The listing builds one solid part. Answer for the finished solid, in the listing's coordinates (mm). Coordinates: 2 decimals unless noted, no trailing zeros. Loops run counter-clockwise (first coordinate to the right, second up) from the corner with the lowest first, then second, coordinate; pieces in that order, holes last. Notation, with made-up numbers: M 2.25,9.5 L 50.25,9.5 A22 cw 50.25,41.5 Z; hole C 15.25,47 d6. An arc over 180 degrees is marked long. Answer as a JSON object with one key per item and string values. Group by question number.
1. A cutting plane is placed at D-D on x = 25. Give the vertices of the cut face in (y, z).
2. A cutting plane is placed at C-C on x = -5. Give the vertices of the cut face in (y, z), and give its area (3 significant figures).
3. Straight lines are drawn through the part: L1, parallel to Y at x = -42.5, z = 1.75; L2, parallel to X at y = -6.5, z = 2.75; L3, parallel to Y at x = -45, z = 0.45. For each, find the intervals that lie inside material, in ascending order.
4. Given pin 1 (1.5 mm diameter, centred on y = -7, z = 1.5, fed in from -X); pin 2 (1.5 mm diameter, centred on y = -7.5, z = 1, fed in from +X), each flat-ended and moving along its own axis, determine where each tip first touches the part or whether it passes through.
5. A cutting plane is placed at A-A on z = 0.8. State how many separate pieces and enclosed holes the cut face has, and give its area (3 significant figures).
6. A cutting plane is placed at B-B on x = -49.5. Give the vertices of the cut face in (y, z), and give its area (3 significant figures).
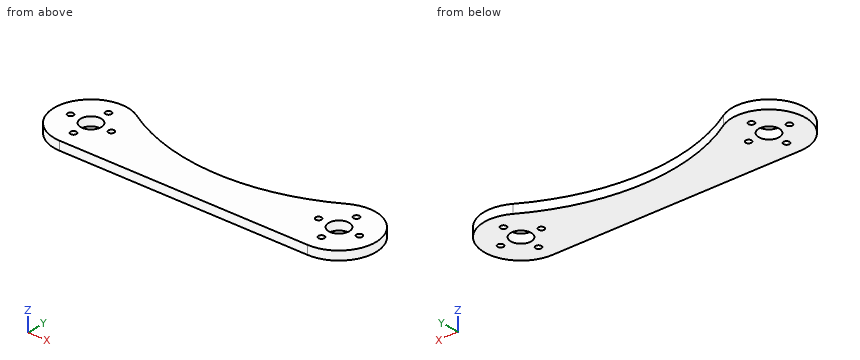
from build123d import *

# Parameters (mm, degrees)
SKETCH1_R           = 3.5
SKETCH1_R_2         = 1
BOSS_EXTRUDE1_DEPTH = 3


with BuildPart() as part:
    # Sketch1 → Boss-Extrude1 (new body)
    with BuildSketch(Plane.XY):
        with BuildLine():
            Line((-42.5, -12.5), (42.5, -12.5))
            ThreePointArc((42.5, -12.5), (54.545159585, 3.341276787), (36.060606061, 10.713739109))
            ThreePointArc((36.060606061, 10.713739109), (0, 0.710678119), (-36.060606061, 10.713739109))
            ThreePointArc((-36.060606061, 10.713739109), (-54.545159585, 3.341276787), (-42.5, -12.5))
        make_face()
        with Locations((-42.5, 0)):
            Circle(SKETCH1_R, mode=Mode.SUBTRACT)
        with Locations((42.5, 0)):
            Circle(SKETCH1_R, mode=Mode.SUBTRACT)
        with Locations((-42.5, 7)):
            Circle(SKETCH1_R_2, mode=Mode.SUBTRACT)
        with Locations((-35.5, 0)):
            Circle(SKETCH1_R_2, mode=Mode.SUBTRACT)
        with Locations((-42.5, -7)):
            Circle(SKETCH1_R_2, mode=Mode.SUBTRACT)
        with Locations((-49.5, 0)):
            Circle(SKETCH1_R_2, mode=Mode.SUBTRACT)
        with Locations((42.5, 7)):
            Circle(SKETCH1_R_2, mode=Mode.SUBTRACT)
        with Locations((35.5, 0)):
            Circle(SKETCH1_R_2, mode=Mode.SUBTRACT)
        with Locations((42.5, -7)):
            Circle(SKETCH1_R_2, mode=Mode.SUBTRACT)
        with Locations((49.5, 0)):
            Circle(SKETCH1_R_2, mode=Mode.SUBTRACT)
    extrude(amount=BOSS_EXTRUDE1_DEPTH)


solid = part.part
From the geometry:
{
 "1": {"outline": "M -12.5,0 L 5.33,0 L 5.33,3 L -12.5,3 Z"},
 "2": {"outline": "M -12.5,0 L 0.89,0 L 0.89,3 L -12.5,3 Z", "area": "40.2 mm²"},
 "3": {"L1": "y = -12.5 to -8, -6 to -3.5, 3.5 to 6, 8 to 12.5", "L2": "x = -53.18 to -43.37, -41.63 to 41.63, 43.37 to 53.18", "L3": "y = -12.25 to -2.45, 2.45 to 12.25"},
 "4": {"pin 1": "stops at x = -53.33", "pin 2": "stops at x = 53.02"},
 "5": {"separate pieces": "1", "enclosed holes": "10", "area": "1,890 mm²"},
 "6": {"outline": "M -10.36,0 L -1,0 L -1,3 L -10.36,3 Z; M 1,0 L 10.36,0 L 10.36,3 L 1,3 Z", "area": "56.1 mm²"}
}
